Read the model definition and answer for the solid it produces. Units are mm, in the model's axes. Face numbers are marked on the shaded views. A direction names the side the tool comes from. Give positions to 0.01 mm unless a question says otherwise; leave off trailing zeros. Write each loop counter-clockwise with the first axis right and the second up, starting at its lowest first coordinate (ties: lowest second). Pieces come first, ordered by that corner, then holes. Notation, with made-up numbers: (86, -3.75) - (92, -3.75) arc R24 cw to (92, 20.25) - close; hole circle Ø11 at (-28.75, 10). An arc over 180 degrees is marked (long way). Answer as CSV lines item,"result".
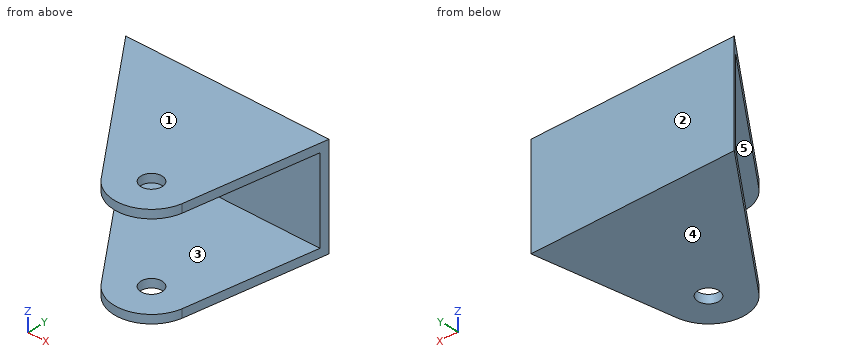
```python
from build123d import *

# Parameters (mm, degrees)
F1_DEPTH = 30.48
F2_T     = -2.54
F4_D     = 6.35


with BuildPart() as f1:
    # F0 (on Top) → F1 (new body)
    with BuildSketch(Plane.XY):
        with BuildLine():
            Line((28.424608, 4.662237), (35.055646, 45.632264))
            Line((35.055646, 45.632264), (-25.904354, 45.632264))
            Line((-25.904354, 45.632264), (8.502317, 0))
            ThreePointArc((8.502317, 0), (19.9818, -4.156915), (28.424608, 4.662237))
        make_face()
    extrude(amount=F1_DEPTH)

    # F2
    f2_openings = [f1.faces().sort_by_distance(p)[0] for p in [
        (19.9818, -4.156915, 15.24),
        (31.740127, 25.14725, 15.24),
        (-8.701018, 22.816132, 15.24),
    ]]
    offset(amount=F2_T, openings=f2_openings)

    # F4 (through all)
    with Locations(Plane.XY.offset(30.48)):
        with Locations((17.433136, 6.733826)):
            Hole(F4_D / 2)


solid = f1.part
```
(1) A cutting plane is placed at B-B (y = 35.5). Write down the section's boundary in (x, z).
Worked out:
outline,"(-18.26, 0) - (33.42, 0) - (33.42, 2.54) - (-18.26, 2.54) - close; (-18.26, 27.94) - (33.42, 27.94) - (33.42, 30.48) - (-18.26, 30.48) - close"
(2) A cutting plane is placed at A-A (x = 16). Write down the section's boundary in (y, z), and give its area (3 significant figures).
Worked out:
outline,"(-4.36, 0) - (3.9, 0) - (3.9, 2.54) - (-4.36, 2.54) - close; (-4.36, 27.94) - (3.9, 27.94) - (3.9, 30.48) - (-4.36, 30.48) - close; (9.57, 0) - (45.63, 0) - (45.63, 30.48) - (9.57, 30.48) - (9.57, 27.94) - (43.09, 27.94) - (43.09, 2.54) - (9.57, 2.54) - close"
area,"290 mm^2"
(3) The mould has two halves that part along Z. Classify the marked faces 1, 2 and 3: +Z half, -Z half, draft (parallel to the pull), parting line (faces both ways), or undercut.
Worked out:
face 1,"+Z half"
face 2,"draft"
face 3,"undercut"
(4) A cutting plane is placed at D-D (z = 14.5). Write down the section's boundary in (x, y), and give its area (3 significant figures).
Worked out:
outline,"(-25.9, 45.63) - (-23.99, 43.09) - (34.64, 43.09) - (35.06, 45.63) - close"
area,"152 mm^2"
(5) Find the intervals of material crossed by L1, parallel to Z at x = -3.5, y = 24; L2, parallel to Y at x = 1, z = 11, in increasing order.
Worked out:
L1,"z = 0 to 2.54, 27.94 to 30.48"
L2,"y = 43.09 to 45.63"
(6) For the marked faces 4 and 5, determine the directions among +Z, -Z, +X, -X, +Y, -Y from which every point of the face is accessible in a straight line to the end or side of a thin tool.
Worked out:
face 4,"-Z, +X, -X, +Y, -Y"
face 5,"+X, -X, -Y"
(7) Each of these flat-tipped pins is pushed along its axis until it touches: P1, Ø10, axis at y = 13.5, z = 25, coming from the -X side; P2, Ø10, axis at x = -19, z = 4, coming from the -Y side. Where does it stop, or does it pass through?
Worked out:
P1,"stops at x = -4.73"
P2,"stops at y = 30.13"
(8) A cutting plane is placed at C-C (y = 8). Write down the section's boundary in (x, z).
Worked out:
outline,"(2.47, 0) - (14.52, 0) - (14.52, 2.54) - (2.47, 2.54) - close; (2.47, 27.94) - (14.52, 27.94) - (14.52, 30.48) - (2.47, 30.48) - close; (20.34, 0) - (28.96, 0) - (28.96, 2.54) - (20.34, 2.54) - close; (20.34, 27.94) - (28.96, 27.94) - (28.96, 30.48) - (20.34, 30.48) - close"
